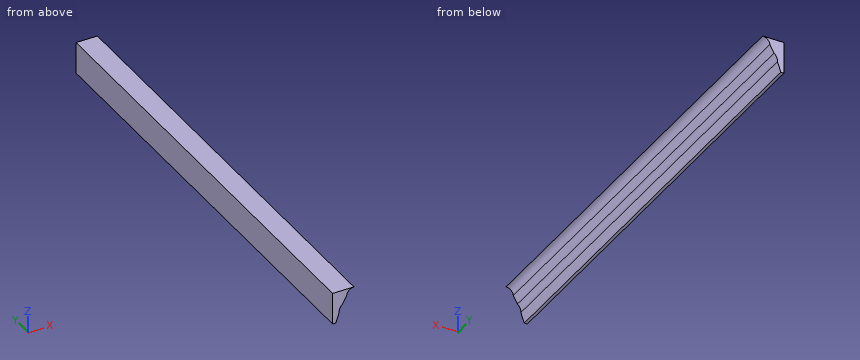
from build123d import *

# Parameters (mm, degrees)
F1_DEPTH = 1092.2


with BuildPart() as f1:
    # F0 (on Front) → F1 (new body, symmetric)
    with BuildSketch(Plane.XZ):
        with BuildLine():
            Line((0, 152.4), (0, 0))
            Line((0, 0), (14.721692, 0))
            Line((14.721692, 0), (30.908439, 47.127715))
            ThreePointArc((30.908439, 47.127715), (34.639248, 67.810302), (46.981968, 84.820464))
            Line((46.981968, 84.820464), (67.011952, 120.723277))
            ThreePointArc((67.011952, 120.723277), (78.149265, 143.284197), (101.6, 152.4))
            Line((101.6, 152.4), (0, 152.4))
        make_face()
    extrude(amount=F1_DEPTH, both=True)


solid = f1.part
Build history of the part. All positions in model axes, mm. Give positions to 0.01 mm unless a question says otherwise; leave off trailing zeros. Order: outer loops, then holes, each group sorted by start corner. A loop starts at its lowest first (then second) coordinate and runs counter-clockwise, first axis right, second up. Notation, with made-up numbers: M 34,30.5 L 79,30.5 A10 cw 79,37.5 Z; hole C -38,45.5 d5. An arc over 180 degrees is marked long. Put each result on its own line as item: value.
Item 1: Wall check: probe 1 along X at (y, z) = (-460, 53); probe 2 along X at (y, z) = (-839.5, 121); probe 3 along Z at (x, y) = (95, 626). Give the ranges that are in metal, low to high.
Results are:
probe 1: 0 to 31
probe 2: 0 to 67.04
probe 3: 151.77 to 152.4
Item 2: Drop a flat-ended pin along its axis: pin 1 Ø3 at (y, z) = (-872, 60) entering from +X. Give the stop position or say it passes through.
Results are:
pin 1: x = 32.46
Item 3: Cut at B-B on z = 67. Write the cut outline in (x, y).
Results are:
outline: M 0,-1092.2 L 34.3,-1092.2 L 34.3,1092.2 L 0,1092.2 Z
Item 4: Cut at A-A on y = -611. Write the cut outline in (x, z), then the cut area to 3 significant figures.
Results are:
outline: M 0,0 L 14.72,0 L 30.91,47.13 A47.18 cw 46.98,84.82 L 67.01,120.72 A34.72 cw 101.6,152.4 L 0,152.4 Z
area: 6,840 mm2
Item 5: Cut at C-C on x = 86. Write the cut outline in (y, z).
Results are:
outline: M -1092.2,148.7 L 1092.2,148.7 L 1092.2,152.4 L -1092.2,152.4 Z
